Geometry check sheet. Reference: the model listing, model coordinates, mm. Face numbers are marked on the shaded views. A direction names the side the tool comes from. Round coordinates to 2 decimals unless told otherwise and drop trailing zeros. Loops run counter-clockwise (first coordinate to the right, second up) from the corner with the lowest first, then second, coordinate; pieces in that order, holes last.
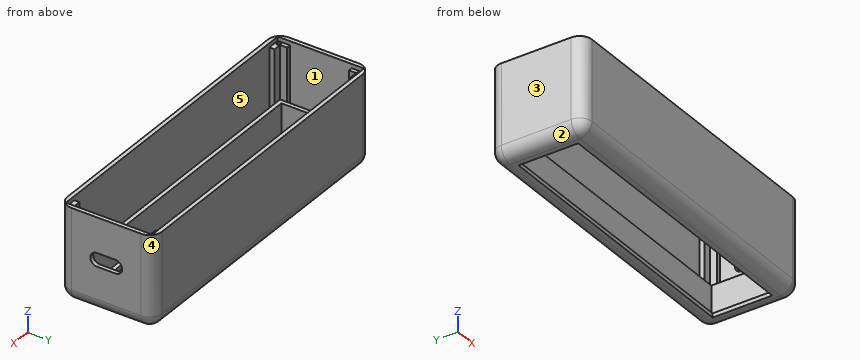
```python
from build123d import *

# Parameters (mm, degrees)
SKETCH_1_W          = 154
SKETCH_1_H          = 46
SKETCH_1_W_2        = 150
SKETCH_1_H_2        = 42
EXTRUDE_1_DEPTH     = 43
SKETCH_2_W          = 154
SKETCH_2_H          = 46
EXTRUDE_2_DEPTH     = 2
SKETCH_3_W          = 137.467290134
SKETCH_3_H          = 29
CUT_EXTRUDE_1_DEPTH = 2
SKETCH_3_4_W        = 146
SKETCH_3_4_H        = 37
SKETCH_3_4_W_2      = 142
SKETCH_3_4_H_2      = 33
EXTRUDE_3_DEPTH     = 15
EXTRUDE_9_DEPTH     = 41
SKETCH_8_R          = 0.95
CUT_EXTRUDE_2_DEPTH = 41
FILLET_2_R          = 6
FILLET_3_R          = 6
CUT_EXTRUDE_3_DEPTH = 41


with BuildPart() as part:
    # 草图1 → 凸台-拉伸1 (new body)
    with BuildSketch(Plane.XY):
        with Locations((1.242355366, -16.575185829)):
            Rectangle(SKETCH_1_W, SKETCH_1_H)
        with Locations((1.242355366, -16.575185829)):
            Rectangle(SKETCH_1_W_2, SKETCH_1_H_2, mode=Mode.SUBTRACT)
    extrude(amount=EXTRUDE_1_DEPTH)

    # 草图2 → 凸台-拉伸2 (add)
    with BuildSketch(Plane(origin=(0, 0, 0), x_dir=(-1, 0, 0), z_dir=(0, 0, -1))):
        with Locations((-1.242355366, -16.575185829)):
            Rectangle(SKETCH_2_W, SKETCH_2_H)
    extrude(amount=EXTRUDE_2_DEPTH)

    # 草图3 → 切除-拉伸1 (cut)
    with BuildSketch(Plane.XY):
        with Locations((1.508710299, -16.575185829)):
            Rectangle(SKETCH_3_W, SKETCH_3_H)
    extrude(amount=-CUT_EXTRUDE_1_DEPTH, mode=Mode.SUBTRACT)

    # 草图3<4> → 凸台-拉伸3 (add)
    with BuildSketch(Plane.XY):
        with Locations((1.242355366, -16.575185829)):
            Rectangle(SKETCH_3_4_W, SKETCH_3_4_H)
        with Locations((1.242355366, -16.575185829)):
            Rectangle(SKETCH_3_4_W_2, SKETCH_3_4_H_2, mode=Mode.SUBTRACT)
    extrude(amount=EXTRUDE_3_DEPTH)

    # 草图7 → 凸台-拉伸9 (add)
    with BuildSketch(Plane.XY):
        Polygon((-73.757644634, 4.424814171), (-67.757644634, 4.424814171), (-67.757644634, 1.924814171), (-71.757644634, 1.924814171), (-71.757644634, -1.575185829), (-73.757644634, -1.575185829), align=None)
        Polygon((74.242355366, -1.575185829), (76.242355366, -1.575185829), (76.242355366, 4.424814171), (70.242355366, 4.424814171), (70.242355366, 1.924814171), (74.242355366, 1.924814171), align=None)
        Polygon((74.242355366, -35.075185829), (74.242355366, -31.575185829), (76.242355366, -31.575185829), (76.242355366, -37.575185829), (70.242355366, -37.575185829), (70.242355366, -35.075185829), align=None)
        Polygon((-71.757644634, -31.575185829), (-73.757644634, -31.575185829), (-73.757644634, -37.575185829), (-67.757644634, -37.575185829), (-67.757644634, -35.075185829), (-71.757644634, -35.075185829), align=None)
    extrude(amount=EXTRUDE_9_DEPTH)

    # 草图8 → 切除-拉伸2 (cut)
    with BuildSketch(Plane.XY.offset(41)):
        with Locations((-72.257644634, 2.924814171)):
            Circle(SKETCH_8_R)
        with Locations((-72.257644634, -36.075185829)):
            Circle(SKETCH_8_R)
        with Locations((74.742355366, -36.075185829)):
            Circle(SKETCH_8_R)
        with Locations((74.742355366, 2.924814171)):
            Circle(SKETCH_8_R)
    extrude(amount=-CUT_EXTRUDE_2_DEPTH, mode=Mode.SUBTRACT)

    # 圆角2
    fillet_2_edges = [part.edges().sort_by_distance(p)[0] for p in [
        (-75.757644634, 6.424814171, 20.5),
        (78.242355366, 6.424814171, 20.5),
        (78.242355366, -39.575185829, 20.5),
        (-75.757644634, -39.575185829, 20.5),
    ]]
    fillet(fillet_2_edges, radius=FILLET_2_R)

    # 圆角3
    fillet_3_edges = [part.edges().sort_by_distance(p)[0] for p in [
        (78.242355366, -16.575185829, -2),
        (1.242355366, -39.575185829, -2),
        (-75.757644634, -16.575185829, -2),
        (1.242355366, 6.424814171, -2),
        (-74.000285321, 4.667454858, -2),
        (-74.000285321, -37.817826516, -2),
        (76.484996053, 4.667454858, -2),
        (76.484996053, -37.817826516, -2),
    ]]
    fillet(fillet_3_edges, radius=FILLET_3_R)

    # 草图12 → 切除-拉伸3 (cut)
    with BuildSketch(Plane.ZY.offset(-76.242355366)):
        with BuildLine():
            Line((26.061737121, -12.075185829), (26.061737121, -21.075185829))
            ThreePointArc((26.061737121, -21.075185829), (22.811737121, -24.325185829), (19.561737121, -21.075185829))
            Line((19.561737121, -21.075185829), (19.561737121, -12.075185829))
            ThreePointArc((19.561737121, -12.075185829), (22.811737121, -8.825185829), (26.061737121, -12.075185829))
        make_face()
    extrude(amount=-CUT_EXTRUDE_3_DEPTH, mode=Mode.SUBTRACT)


solid = part.part
```
1) Mould release check, pull along X, two halves, no side actions. Record for the marked faces 3, 4 and 5: +X half, -X half, draft (parallel to the pull), parting line (faces both ways), or undercut.
Report:
face 3: -X half
face 4: +X half
face 5: undercut
2) Access from +Z, -Z, +X, -X, +Y, -Y to the whole of each face (thin tool, end or side, straight path). Record for the marked faces 1 and 2.
Report:
face 1: +Z
face 2: -Z, -X, +Y, -Y
3) Scan lines: line 1 along X through (y, z) = (-20.5, 9); line 2 along Y through (x, z) = (26, 4); line 3 along Y through (x, z) = (18.5, 32.5). Record each from-to range of solid material in increasing order.
Report:
line 1: x = -75.76 to -73.76, -71.76 to -69.76, 72.24 to 74.24, 76.24 to 78.24
line 2: y = -39.58 to -37.58, -35.08 to -33.08, -0.08 to 1.92, 4.42 to 6.42
line 3: y = -39.58 to -37.58, 4.42 to 6.42
4) Sectioned sample at C-C, the plane z = 5.5. State how many separate pieces and enclosed holes the cut face has, then the cut area to 3 significant figures.
Report:
separate pieces: 1
enclosed holes: 9
area: 1,550 mm2
5) Sectioned sample at B-B, the plane y = -28.5. Record the cut outline in (x, z), then the cut area to 3 significant figures.
Report:
outline: (-75.76, 4) arc R6 ccw to (-69.76, -2) - (-67.22, -2) - (-67.22, 0) - (-69.76, 0) - (-69.76, 15) - (-71.76, 15) - (-71.76, 0) - (-73.76, 0) - (-73.76, 43) - (-75.76, 43) - close; (70.24, -2) - (72.24, -2) arc R6 ccw to (78.24, 4) - (78.24, 43) - (76.24, 43) - (76.24, 0) - (74.24, 0) - (74.24, 15) - (72.24, 15) - (72.24, 0) - (70.24, 0) - close
area: 250 mm2
6) Gauge pin test, flat ends, axial feed: pin 1 (2 mm diameter, centred on x = -73, z = 28, fed in from +Y); pin 2 (6.5 mm diameter, centred on x = -70, y = 1, fed in from +Z); pin 3 (1 mm diameter, centred on x = 21, z = 2.5, fed in from -Y). Record the tip position at first contact, or that the pin passes through.
Report:
pin 1: stops at y = 5.99
pin 2: stops at z = 41
pin 3: stops at y = -39.49
7) Sectioned sample at A-A, the plane x = 44. Record the cut outline in (y, z).
Report:
outline: (-39.58, 4) arc R6 ccw to (-33.58, -2) - (-31.08, -2) - (-31.08, 0) - (-33.08, 0) - (-33.08, 15) - (-35.08, 15) - (-35.08, 0) - (-37.58, 0) - (-37.58, 43) - (-39.58, 43) - close; (-2.08, -2) - (0.42, -2) arc R6 ccw to (6.42, 4) - (6.42, 43) - (4.42, 43) - (4.42, 0) - (1.92, 0) - (1.92, 15) - (-0.08, 15) - (-0.08, 0) - (-2.08, 0) - close
